Print and shaded views of the part. All mm, measured from the part's lowest x, y and z. A direction names the side the tool comes from. Give positions to 0.01 mm unless a question says otherwise; leave off trailing zeros. Write each loop counter-clockwise with the first axis right and the second up, starting at its lowest first coordinate (ties: lowest second). Pieces come first, ordered by that corner, then holes. Notation, with made-up numbers: M 71.5,9.5 L 78.5,9.5 A26 cw 78.5,33.5 Z; hole C 17.5,75.5 d11. An arc over 180 degrees is marked long. One line per question, with ' | ' between items. Start each with the question number.
1. Cut at A-A, the plane x = 54. Write the cut outline in (y, z).
2. Flat gauge pins, fed straight in: pin 1 (6 mm diameter, centred on x = 90.5, y = 18, fed in from -Z) (1 decimal); pin 2 (6 mm diameter, centred on y = 14.5, z = 47, fed in from +X). Where does each tip first touch, or does it go through?
3. Cut at C-C, the plane y = 46.5. Write the cut outline in (x, z) (1 decimal), then the cut area to 3 significant figures.
4. Wall check: L1, parallel to Z at x = 54, y = 23; L2, parallel to X at y = 46, z = 40.5; L3, parallel to X at y = 41.5, z = 44. Give the ranges that are in metal, low to high.
5. Which spindle directions (+Z, -Z, +X, -X, +Y, -Y) get a long thin tool onto all of the face, cutting with end or side? Do the marked faces 1 and 2. Say none if no direction does.
6. Cut at B-B, the plane z = 59. Write the cut outline in (x, y) (1 decimal).
7. Cut at D-D, the plane z = 18. Write the cut outline in (x, y).
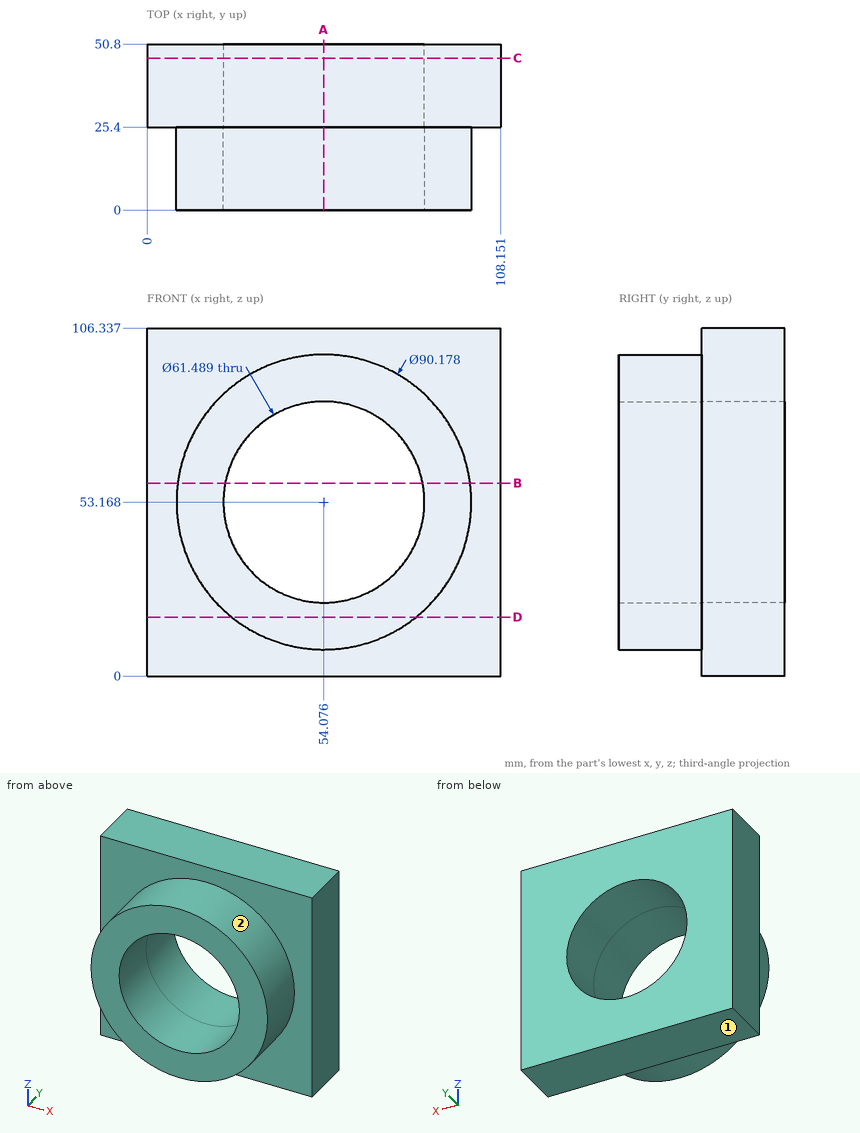
Here are the results:
1) outline: M 0,8.08 L 25.4,8.08 L 25.4,0 L 50.8,0 L 50.8,22.42 L 0,22.42 Z; M 0,83.91 L 50.8,83.91 L 50.8,106.34 L 25.4,106.34 L 25.4,98.26 L 0,98.26 Z
2) pin 1: z = 22.9 | pin 2: x = 99.05
3) outline: M 0,0 L 108.2,0 L 108.2,106.3 L 0,106.3 Z; hole C 54.1,53.2 d61.5 | area: 8,530 mm^2
4) L1: 8.08 to 22.42, 83.91 to 98.26 | L2: 0 to 26.06, 82.09 to 108.15 | L3: 0 to 24.73, 83.42 to 108.15
5) face 1: -Z, +X, -X, +Y, -Y | face 2: -Y
6) outline: M 0,25.4 L 9.4,25.4 L 9.4,0 L 23.9,0 L 23.9,50.8 L 0,50.8 Z; M 84.3,0 L 98.8,0 L 98.8,25.4 L 108.2,25.4 L 108.2,50.8 L 84.3,50.8 Z
7) outline: M 0,25.4 L 25.86,25.4 L 25.86,0 L 82.29,0 L 82.29,25.4 L 108.15,25.4 L 108.15,50.8 L 0,50.8 Z
